```python
from build123d import *

# Parameters (mm, degrees)
SKETCH001_R       = 0.45
PAD001_DEPTH      = 6.5
PAD001_DEPTH_BACK = 3.5
SKETCH_R          = 6
PAD_DEPTH         = 13
FILLET_R          = 0.5


with BuildPart() as pad001:
    # Sketch001 → Pad001 (new body, two sides)
    with BuildSketch(Plane.XY.offset(0.5)) as pad001_sk:
        Circle(SKETCH001_R)
        with Locations((10, 0)):
            Circle(SKETCH001_R)
    extrude(amount=PAD001_DEPTH)
    extrude(pad001_sk.sketch, amount=-PAD001_DEPTH_BACK)


with BuildPart() as obj1:
    # Sketch → Pad (new body)
    with BuildSketch(Plane.XY.offset(0.1)):
        with Locations((5, 0)):
            Circle(SKETCH_R)
    extrude(amount=PAD_DEPTH)

    # Fillet
    fillet_edges = [obj1.edges().sort_by_distance(p)[0] for p in [
        (-1, 0, 0.1),
        (-1, 0, 13.1),
    ]]
    fillet(fillet_edges, radius=FILLET_R)

    # obj1: union Pad001
    add(pad001.part)


solid = obj1.part
```
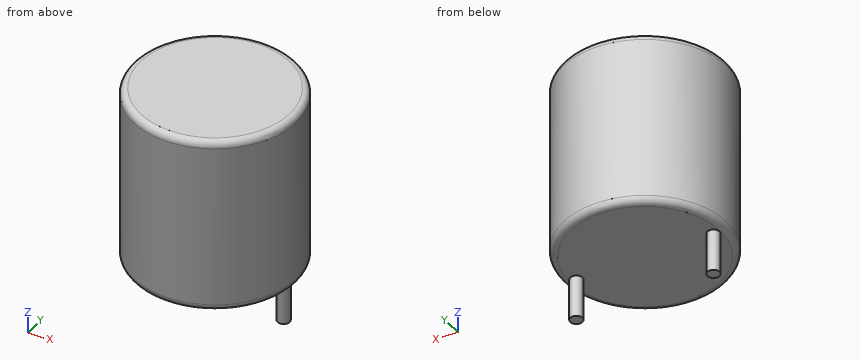
Source: CAD feature listing. Evaluate the final solid. Frame: model axes, mm. Round coordinates to 2 decimals unless told otherwise and drop trailing zeros. Loops run counter-clockwise (first coordinate to the right, second up) from the corner with the lowest first, then second, coordinate; pieces in that order, holes last. Notation, with made-up numbers: M -10,57.25 L 46,57.25 A33 cw 46,88.25 Z; hole C -10.75,24 d10. An arc over 180 degrees is marked long. Use a Markdown table: item, result. Add a question column.
1. Contact query for flat-ended pins moving along their axis: P1, Ø2, axis at y = 4.5, z = 4.5, coming from the +X side; P2, Ø3, axis at y = 4, z = 11, coming from the +X side; P3, Ø3.5, axis at x = 4.5, y = 2, coming from the -Z side. Output: stop coordinate, or through.
2. Section query B-B on z = 11.75. Return the cut outline in (x, y), then the cut area to 3 significant figures.
3. Line query: line 1 (Z direction, x = 4.5, y = -3); line 2 (Y direction, x = 4.5, z = 6.25); line 3 (X direction, y = 4, z = 2.25). Output: solid intervals per line, ascending.
4. Section query A-A on y = 0. Return the cut outline in (x, z), then the cut area to 3 significant figures.
Reported:
| question | item | result |
|---|---|---|
| 1 | P1 | stops at x = 9.87 |
| 1 | P2 | stops at x = 10.45 |
| 1 | P3 | stops at z = 0.1 |
| 2 | outline | C 5,0 d12 |
| 2 | area | 113 mm² |
| 3 | line 1 | z = 0.1 to 13.1 |
| 3 | line 2 | y = -5.98 to 5.98 |
| 3 | line 3 | x = 0.53 to 9.47 |
| 4 | outline | M -1,0.6 A0.5 ccw -0.5,0.1 L -0.45,0.1 L -0.45,-3 L 0.45,-3 L 0.45,0.1 L 9.55,0.1 L 9.55,-3 L 10.45,-3 L 10.45,0.1 L 10.5,0.1 A0.5 ccw 11,0.6 L 11,12.6 A0.5 ccw 10.5,13.1 L -0.5,13.1 A0.5 ccw -1,12.6 Z |
| 4 | area | 161 mm² |
